Source: CAD feature listing. Evaluate the final solid. Frame: model axes, mm. Face numbers are marked on the shaded views. A direction names the side the tool comes from. Coordinates: 2 decimals unless noted, no trailing zeros. Order: outer loops, then holes, each group sorted by start corner. A loop starts at its lowest first (then second) coordinate and runs counter-clockwise, first axis right, second up.
Item 1: Section A-A on z = 0. Return the cut outline in (x, y), then the cut area to 3 significant figures.
Item 2: Section C-C on y = 48.5. Return the cut outline in (x, z), then the cut area to 3 significant figures.
Item 3: Reachability of the marked faces 1 and 2 from +Z, -Z, +X, -X, +Y, -Y: full face, straight path, thin tool, end or side. Return the list, or none.
Item 4: Ray query, line 1 (Y direction, x = 35, z = -37.5); line 2 (X direction, y = 13.5, z = -1); line 3 (X direction, y = 45.5, z = -50). Return the intervals inside material, ascending.
Item 5: Contact query for flat-ended pins moving along their axis: P1, Ø1, axis at x = -48.5, z = -0.5, coming from the +Y side; P2, Ø10, axis at x = 0, z = -50, coming from the +Y side; P3, Ø1.5, axis at x = 39.5, y = 21, coming from the -Z side (3 decimals). Output: stop coordinate, or through.
Item 6: Section B-B on y = 8. Return the cut outline in (x, z), then the cut area to 3 significant figures.
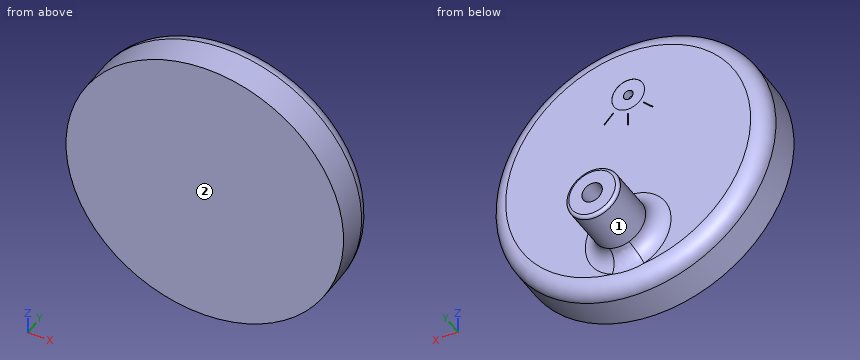
from build123d import *

# Parameters (mm, degrees)
SKETCH1_R           = 85
BOSS_EXTRUDE1_DEPTH = 30
FILLET1_R           = 10
SHELL1_T            = -8
SKETCH1_2_R         = 85
BOSS_EXTRUDE3_DEPTH = 5
SKETCH2_R           = 16.25
SKETCH2_R_2         = 6.25
BOSS_EXTRUDE2_DEPTH = 40
CUT_EXTRUDE1_REACH  = 128.689
SKETCH2_3_R         = 6.25
FILLET2_R           = 10
FILLET3_R           = 2
SKETCH3_R           = 3
CUT_EXTRUDE2_DEPTH  = 5
SKETCH4_R           = 10
SKETCH4_W           = 0.5
SKETCH4_H           = 8
CUT_EXTRUDE3_DEPTH  = 0.1


with BuildPart() as part:
    # Sketch1 → Boss-Extrude1 (new body)
    with BuildSketch(Plane(origin=(0, 0, 0), x_dir=(1, 0, 0), z_dir=(0, 1, 0))):
        with Locations(Location((0, 0, 0), (0, 0, 270))):
            Circle(SKETCH1_R)
    extrude(amount=BOSS_EXTRUDE1_DEPTH)

    # Fillet1
    fillet1_edges = [part.edges().sort_by_distance(p)[0] for p in [
        (0, 30, -85),
    ]]
    fillet(fillet1_edges, radius=FILLET1_R)

    # Shell1
    shell1_openings = [part.faces().sort_by_distance(p)[0] for p in [
        (0, 0, 0),
    ]]
    offset(amount=SHELL1_T, openings=shell1_openings, kind=Kind.INTERSECTION)

    # Sketch1_2 → Boss-Extrude3 (add)
    with BuildSketch(Plane(origin=(0, 0, 0), x_dir=(1, 0, 0), z_dir=(0, 1, 0))):
        with Locations(Location((0, 0, 0), (0, 0, 270))):
            Circle(SKETCH1_2_R)
    extrude(amount=BOSS_EXTRUDE3_DEPTH)

    # Sketch2 → Boss-Extrude2 (add)
    with BuildSketch(Plane(origin=(0, 30, 0), x_dir=(1, 0, 0), z_dir=(0, 1, 0))):
        with Locations(Location((0, 50, 0), (0, 0, 270))):
            Circle(SKETCH2_R)
        with Locations(Location((0, 50, 0), (0, 0, 270))):
            Circle(SKETCH2_R_2, mode=Mode.SUBTRACT)
    extrude(amount=BOSS_EXTRUDE2_DEPTH)

    # Sketch2_3 → Cut-Extrude1 (cut, up to next)
    with BuildSketch(Plane(origin=(0, 30, 0), x_dir=(1, 0, 0), z_dir=(0, 1, 0)), mode=Mode.PRIVATE) as cut_extrude1_sk1:
        with Locations(Location((0, 50, 0), (0, 0, 270))):
            Circle(SKETCH2_3_R)
    cut_extrude1_tool1 = extrude(cut_extrude1_sk1.sketch, amount=-CUT_EXTRUDE1_REACH, mode=Mode.PRIVATE) & part.part
    add(cut_extrude1_tool1.solids().sort_by_distance((0, 30, -50))[0], mode=Mode.SUBTRACT)

    # Fillet2
    fillet2_edges = [part.edges().sort_by_distance(p)[0] for p in [
        (0, 30, -66.25),
    ]]
    fillet(fillet2_edges, radius=FILLET2_R)

    # Fillet3
    fillet3_edges = [part.edges().sort_by_distance(p)[0] for p in [
        (0, 70, -66.25),
    ]]
    fillet(fillet3_edges, radius=FILLET3_R)

    # Sketch3 → Cut-Extrude2 (cut)
    with BuildSketch(Plane(origin=(0, 30, 0), x_dir=(1, 0, 0), z_dir=(0, 1, 0))):
        with Locations(Location((0, -45.554448546, 0), (0, 0, 270))):
            Circle(SKETCH3_R)
    extrude(amount=-CUT_EXTRUDE2_DEPTH, mode=Mode.SUBTRACT)

    # Sketch4 → Cut-Extrude3 (cut)
    with BuildSketch(Plane(origin=(0, 30, 0), x_dir=(1, 0, 0), z_dir=(0, 1, 0))):
        with Locations(Location((0, -45.718475917, 0), (0, 0, 270))):
            Circle(SKETCH4_R)
        Polygon((8.929220054, -36.270245709), (9.292745114, -36.613537902), (14.78542021, -30.797136927), (14.421895149, -30.453844734), align=None)
        with Locations((0.080103939, -28.718475917)):
            Rectangle(SKETCH4_W, SKETCH4_H)
        Polygon((-9.280005487, -36.611116357), (-9.623297681, -36.974641418), (-15.439698655, -31.481966322), (-15.096406462, -31.118441261), align=None)
    extrude(amount=-CUT_EXTRUDE3_DEPTH, mode=Mode.SUBTRACT)


solid = part.part
Answer list:
1. outline: (-85, 0) - (85, 0) - (85, 20) arc R10 ccw to (75, 30) - (-75, 30) arc R10 ccw to (-85, 20) - close; hole (-77, 5) - (77, 5) - (77, 20) arc R2 ccw to (75, 22) - (-75, 22) arc R2 ccw to (-77, 20) - close
1. area: 2,440 mm2
2. outline: circle Ø32.5 at (0, -50); hole circle Ø12.5 at (0, -50)
2. area: 707 mm2
3. face 1: +Y
3. face 2: +Z, -Z, +X, -X, -Y
4. line 1: y = 0 to 5, 22 to 30
4. line 2: x = -84.99 to -76.99, 76.99 to 84.99
4. line 3: x = -16.25 to -6.25, 6.25 to 16.25
5. P1: stops at y = 30
5. P2: stops at y = 5
5. P3: stops at z = -75.605
6. outline: circle Ø170 at (0, 0); hole circle Ø154 at (0, 0)
6. area: 4,070 mm2
